Part print with two shaded views. Sizes in mm from the minimum x, y, z corner. A direction names the side the tool comes from. Round coordinates to 2 decimals unless told otherwise and drop trailing zeros. Write each loop counter-clockwise with the first axis right and the second up, starting at its lowest first coordinate (ties: lowest second). Pieces come first, ordered by that corner, then holes. Notation, with made-up numbers: M 58,-27.75 L 104,-27.75 A30 ccw 104,8.25 Z; hole C -13.75,57 d2. An arc over 180 degrees is marked long. One line per question, with ' | ' between items. Start each with the question number.
1) Mould opens along X. For the marked faces 1, 2 and 3 say: pulls with the +X half, pulls with the -X half, needs draft (parallel to the pull), parting line crosses it, or undercut.
2) Saw through at C-C (z = 6). List the corners of the cut face in (x, y).
3) Wall check: probe 1 along X at (y, z) = (1.9, 5); probe 2 along Z at (x, y) = (18, 2.05); probe 3 along Z at (x, y) = (3, 1.05) (1 decimal). Give the ranges that are in metal, low to high. Write a range as [from, to].
4) Saw through at D-D (x = 18.5). List the corners of the cut face in (y, z), plus the area to 3 significant figures.
5) Drop flat-ended pins along their axis: pin 1 Ø1.5 at (x, y) = (17, 1) entering from +Z; pin 2 Ø3 at (x, z) = (25, 5) entering from +Y; pin 3 Ø6.5 at (x, z) = (5, 5) entering from -Y. Give the stop position or say it passes through.
6) Tool access for the marked faces 4 and 5: list every direction of +Z, -Z, +X, -X, +Y, -Y with a clear straight run to the whole face (end or side of a thin tool).
7) Saw through at A-A (y = 2.3). List the corners of the cut face in (x, z) (1 decimal).
8) Saw through at B-B (x = 26.5). List the corners of the cut face in (y, z).
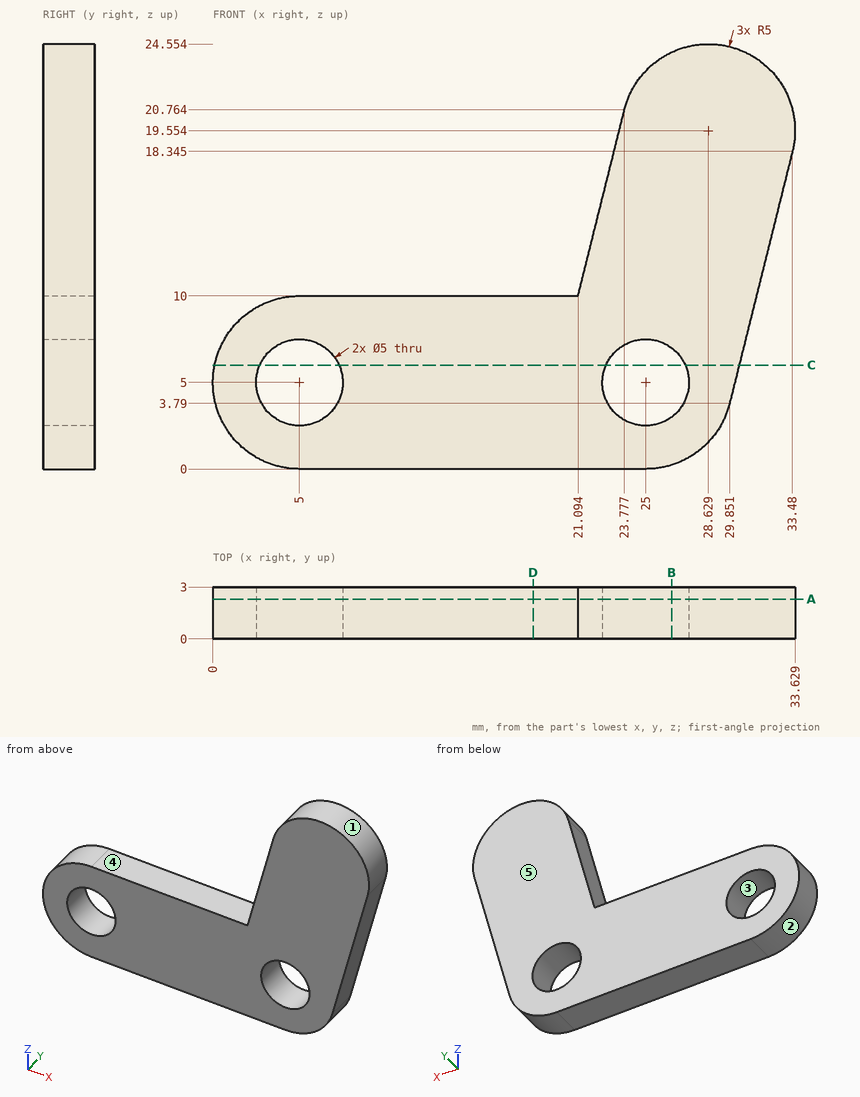
Answer key:
1) face 1: parting line crosses it | face 2: pulls with the -X half | face 3: undercut
2) outline: M 0.1,0 L 2.71,0 L 2.71,3 L 0.1,3 Z; M 7.29,0 L 22.71,0 L 22.71,3 L 7.29,3 Z; M 27.29,0 L 30.4,0 L 30.4,3 L 27.29,3 Z
3) probe 1: x = [0, 2.5], [7.5, 22.5], [27.5, 30.15] | probe 2: z = [0, 10] | probe 3: z = [0.4, 3.5], [6.5, 9.6]
4) outline: M 0,0 L 3,0 L 3,10 L 0,10 Z | area: 30.0 mm2
5) pin 1: stops at z = 10 | pin 2: passes through | pin 3: stops at y = 0
6) face 4: +Z, -X, +Y, -Y | face 5: +Z, -Z, +X, -X, +Y
7) outline: M 5,0 L 25,0 A5 ccw 29.9,3.8 L 33.5,18.3 A5 ccw 23.8,20.8 L 21.1,10 L 5,10 A5 ccw Z; hole C 5,5 d5; hole C 25,5 d5
8) outline: M 0,0.23 L 3,0.23 L 3,3 L 0,3 Z; M 0,7 L 3,7 L 3,24.08 L 0,24.08 Z
